from build123d import *

# Parameters (mm, degrees)
SCHIZZO2_W                   = 100
SCHIZZO2_H                   = 10
ESTRUSIONE_ESTRUSIONE1_DEPTH = 78
SCHIZZO3_R                   = 2
TAGLIO_ESTRUSIONE1_DEPTH     = 15
TAGLIO_ESTRUSIONE2_START     = -15
SCHIZZO4_R                   = 2
TAGLIO_ESTRUSIONE2_DEPTH     = 15


with BuildPart() as part:
    # Schizzo2 → Estrusione-Estrusione1 (new body)
    with BuildSketch(Plane.XY):
        with Locations((50, 5)):
            Rectangle(SCHIZZO2_W, SCHIZZO2_H)
    extrude(amount=-ESTRUSIONE_ESTRUSIONE1_DEPTH)

    # Schizzo3 → Taglio-Estrusione1 (cut)
    with BuildSketch(Plane.XY):
        with Locations((19.5, 5)):
            Circle(SCHIZZO3_R)
        with Locations((50, 5)):
            Circle(SCHIZZO3_R)
        with Locations(Location((80.5, 5, 0), (0, 0, 180))):
            Circle(SCHIZZO3_R)
    extrude(amount=-TAGLIO_ESTRUSIONE1_DEPTH, mode=Mode.SUBTRACT)

    # Schizzo4 → Taglio-Estrusione2 (cut)
    with BuildSketch(Plane(origin=(0, 0, -78), x_dir=(-1, 0, 0), z_dir=(0, 0, -1)).offset(TAGLIO_ESTRUSIONE2_START)):
        with Locations((-80.5, 5)):
            Circle(SCHIZZO4_R)
        with Locations(Location((-50, 5, 0), (0, 0, 180))):
            Circle(SCHIZZO4_R)
        with Locations(Location((-19.5, 5, 0), (0, 0, 180))):
            Circle(SCHIZZO4_R)
    extrude(amount=TAGLIO_ESTRUSIONE2_DEPTH, mode=Mode.SUBTRACT)


solid = part.part
Work out the finished part from the listing and answer in its coordinate system (mm). A direction names the side the tool comes from. Round coordinates to 2 decimals unless told otherwise and drop trailing zeros. Write each loop counter-clockwise with the first axis right and the second up, starting at its lowest first coordinate (ties: lowest second). Pieces come first, ordered by that corner, then holes.
1) Straight lines are drawn through the part: line 1 (Y direction, x = 80.5, z = -68); line 2 (Y direction, x = 19, z = -68); line 3 (Z direction, x = 79, y = 6). For each, find the intervals that lie inside material, in ascending order.
2) The mould has two halves that part along Y. Classify faces 4 (the flat face through (49, 10, -38)), 5 (the cylindrical face through (51.908, 5.601, -7.395)), 6 (the flat face through (49, 3, 0)), 7 (the flat face through (81, 5, -63)): pulls with the +Y half, pulls with the -Y half, needs draft (parallel to the pull), parting line crosses it, or undercut.
3) A cutting plane is placed at B-B (x = 19.5). Give the vertices of the cut face in (y, z).
4) Given pin 1 Ø1 at (y, z) = (7.5, -39.5) entering from -X; pin 2 Ø3 at (x, y) = (80.5, 5) entering from +Z; pin 3 Ø1.2 at (x, y) = (49, 4.5) entering from -Z, each flat-ended and moving along its own axis, determine where each tip first touches the part or whether it passes through.
5) A cutting plane is placed at A-A (y = 5). Give the vertices of the cut face in (x, z), plus the area to 3 significant figures.
6) A tool of negligible diameter and unlimited length cuts with its end or side. For faces 1 (the flat face through (0, 5, -38)), 2 (the flat face through (50, 5, -63)), 3 (the flat face through (81, 5, -15)), from which of +Z, -Z, +X, -X, +Y, -Y can it reach the whole face along a straight path? Write none if from no direction.
Completed:
1. line 1: y = 0 to 3, 7 to 10
1. line 2: y = 0 to 3.06, 6.94 to 10
1. line 3: z = -63 to -15
2. face 4: pulls with the +Y half
2. face 5: undercut
2. face 6: needs draft
2. face 7: undercut
3. outline: (0, -78) - (3, -78) - (3, -63) - (7, -63) - (7, -78) - (10, -78) - (10, 0) - (7, 0) - (7, -15) - (3, -15) - (3, 0) - (0, 0) - close
4. pin 1: stops at x = 0
4. pin 2: stops at z = -15
4. pin 3: stops at z = -63
5. outline: (0, -78) - (17.5, -78) - (17.5, -63) - (21.5, -63) - (21.5, -78) - (48, -78) - (48, -63) - (52, -63) - (52, -78) - (78.5, -78) - (78.5, -63) - (82.5, -63) - (82.5, -78) - (100, -78) - (100, 0) - (82.5, 0) - (82.5, -15) - (78.5, -15) - (78.5, 0) - (52, 0) - (52, -15) - (48, -15) - (48, 0) - (21.5, 0) - (21.5, -15) - (17.5, -15) - (17.5, 0) - (0, 0) - close
5. area: 7,440 mm2
6. face 1: +Z, -Z, -X, +Y, -Y
6. face 2: -Z
6. face 3: +Z
